Source: three-view drawing plus pictorial views. Frame: mm from the lowest corner of the part. A direction names the side the tool comes from. Give positions to 0.01 mm unless a question says otherwise; leave off trailing zeros. Order: outer loops, then holes, each group sorted by start corner. A loop starts at its lowest first (then second) coordinate and runs counter-clockwise, first axis right, second up. Notation, with made-up numbers: (-19.75, 52) -> (-14.75, 52) arc R15 cw to (-14.75, 61) -> close; hole circle Ø8 at (6, 9.25). An arc over 180 degrees is marked (long way). One line per question, with ' | ' between items.
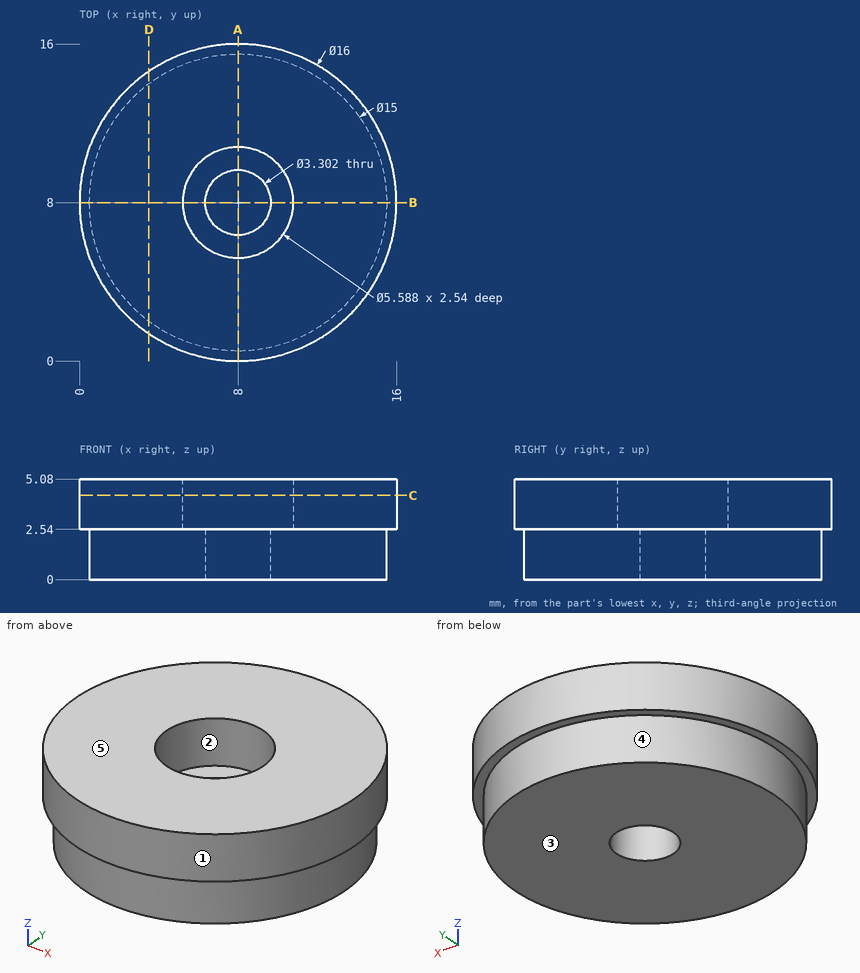
1) Section D-D on x = 3.5. Return loops of the section in (y, z), plus the area to 3 significant figures.
Check result:
outline: (1.39, 2.54) -> (2, 2.54) -> (2, 0) -> (14, 0) -> (14, 2.54) -> (14.61, 2.54) -> (14.61, 5.08) -> (1.39, 5.08) -> close | area: 64.1 mm^2
2) Material intervals for probe 1 along Y at (x, z) = (8, 3.2); probe 2 along Y at (x, z) = (8, 1.1); probe 3 along X at (y, z) = (5.75, 4.75), sorted ascending. Write a range as from..to.
Check result:
probe 1: y = 0..5.21, 10.79..16 | probe 2: y = 0.5..6.35, 9.65..15.5 | probe 3: x = 0.32..6.34, 9.66..15.68
3) Pull-direction query (X, two-part tool) for the marked faces 1, 2 and 3; classes: +X half, -X half, draft (parallel to the pull), parting line (faces both ways), or undercut.
Check result:
face 1: parting line | face 2: undercut | face 3: draft
4) Section C-C on z = 4.25. Return loops of the section in (x, y), plus the area to 3 significant figures.
Check result:
outline: circle Ø16 at (8, 8); hole circle Ø5.59 at (8, 8) | area: 177 mm^2
5) Section A-A on x = 8. Return loops of the section in (y, z).
Check result:
outline: (0, 2.54) -> (0.5, 2.54) -> (0.5, 0) -> (6.35, 0) -> (6.35, 2.54) -> (5.21, 2.54) -> (5.21, 5.08) -> (0, 5.08) -> close; (9.65, 0) -> (15.5, 0) -> (15.5, 2.54) -> (16, 2.54) -> (16, 5.08) -> (10.79, 5.08) -> (10.79, 2.54) -> (9.65, 2.54) -> close
6) Set-up query: the marked faces 4 and 5. Return all of +Z, -Z, +X, -X, +Y, -Y with unobstructed straight access to the full face (end or side cutting, diameter ignored); none if empty.
Check result:
face 4: -Z | face 5: +Z, +X, -X, +Y, -Y
7) Contact query for flat-ended pins moving along their axis: pin 1 Ø4 at (x, y) = (3, 9.5) entering from -Z; pin 2 Ø1 at (x, z) = (2.5, 1) entering from +Y; pin 3 Ø1.5 at (y, z) = (9.5, 1) entering from +X; pin 4 Ø2 at (x, z) = (4.5, 4) entering from -Y. Output: stop coordinate, or through.
Check result:
pin 1: stops at z = 0 | pin 2: stops at y = 13.59 | pin 3: stops at x = 15.46 | pin 4: stops at y = 0.4
